Input: dimensioned drawing with shaded views. Units: mm. Origin: part minimum x, y, z. A direction names the side the tool comes from. Give positions to 0.01 mm unless a question says otherwise; leave off trailing zeros. Write each loop counter-clockwise with the first axis right and the second up, starting at its lowest first coordinate (ties: lowest second). Pieces come first, ordered by that corner, then holes. Notation, with made-up numbers: (-7, 16.5) -> (2, 16.5) arc R24 cw to (2, 37.5) -> close; hole circle Ø6 at (42, 56). An arc over 180 degrees is marked (long way). Answer as a JSON object with one key per item and string values. Group by question number.
(1) Section query B-B on z = 12. Output: boundary loops of the cut face in (x, y), plus the area to 3 significant figures.
(2) Material intervals for probe 1 along Y at (x, z) = (4, 9.25); probe 2 along Z at (x, y) = (2.25, 3.75); probe 3 along Z at (x, y) = (1.5, 2.9), sorted ascending.
(3) Section query D-D on x = 4.25. Output: boundary loops of the cut face in (y, z).
(4) Set-up query: the marked faces 1 and 2. Return all of +Z, -Z, +X, -X, +Y, -Y with unobstructed straight access to the full face (end or side cutting, diameter ignored); none if empty.
(5) Section query A-A on y = 1.6. Output: boundary loops of the cut face in (x, z).
(6) Section query C-C on x = 0.75. Output: boundary loops of the cut face in (y, z), plus the area to 3 significant figures.
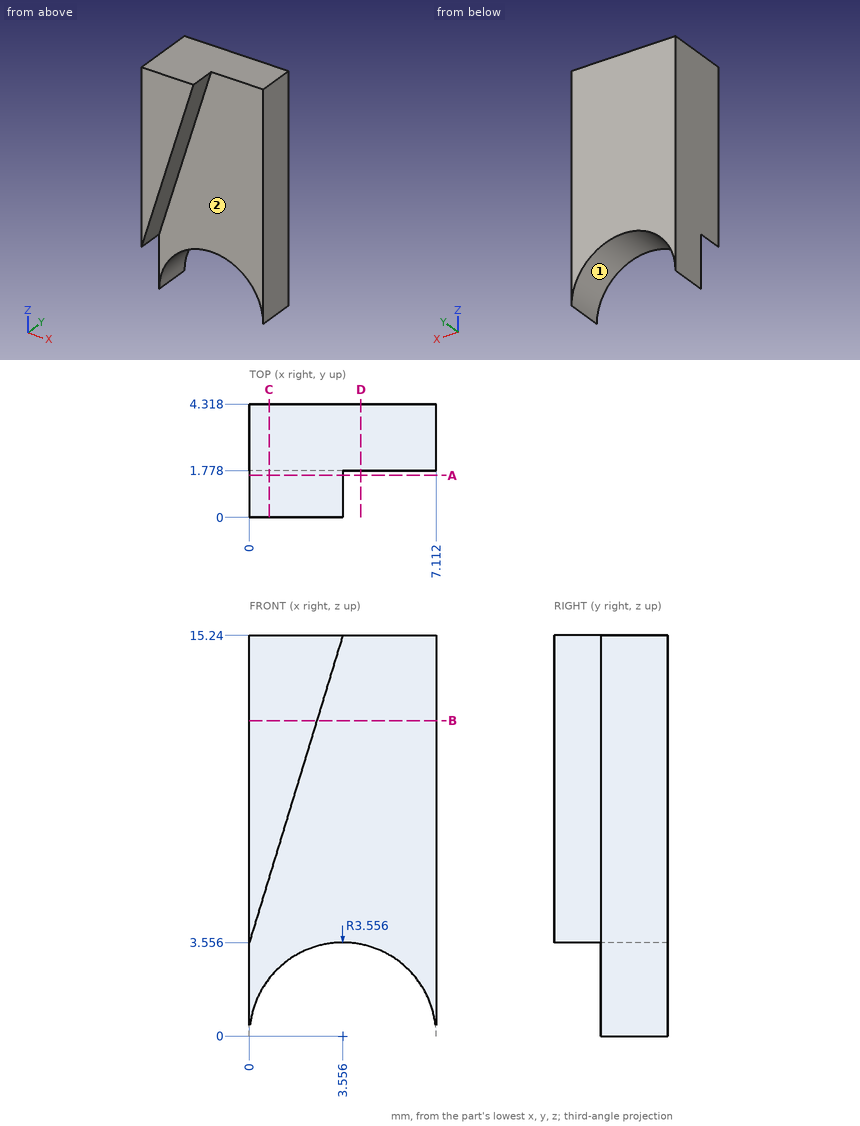
Answer list:
{
 "1": {"outline": "(0, 0) -> (2.57, 0) -> (2.57, 1.78) -> (7.11, 1.78) -> (7.11, 4.32) -> (0, 4.32) -> close", "area": "22.6 mm2"},
 "2": {"probe 1": "1.78 to 4.32", "probe 2": "3.31 to 15.24", "probe 3": "2.9 to 15.24"},
 "3": {"outline": "(1.78, 3.49) -> (4.32, 3.49) -> (4.32, 15.24) -> (1.78, 15.24) -> close"},
 "4": {"face 1": "-Z, +Y, -Y", "face 2": "-Z, +X, -Y"},
 "5": {"outline": "(0, 3.56) -> (3.56, 15.24) -> (0, 15.24) -> close"},
 "6": {"outline": "(0, 6.02) -> (1.78, 6.02) -> (1.78, 2.18) -> (4.32, 2.18) -> (4.32, 15.24) -> (0, 15.24) -> close", "area": "49.6 mm2"}
}
